The figure shows three views and two pictorial views of one solid part (mm, origin at its lowest corner). Answer the questions. A direction names the side the tool comes from. Coordinates: 2 decimals unless noted, no trailing zeros. Loops run counter-clockwise (first coordinate to the right, second up) from the corner with the lowest first, then second, coordinate; pieces in that order, holes last. Notation, with made-up numbers: (21, 75) -> (38, 75) arc R24 ccw to (38, 90) -> close; hole circle Ø6 at (76, -29). An arc over 180 degrees is marked (long way). Answer as a JSON object with one key per item and string values. Group by question number.
1) Which of the six approach directions +Z, -Z, +X, -X, +Y, -Y give full straight-line access (tool end or side, diameter ignored) to the marked faces 1, 2 and 3?
2) Determine the mould class of the marked faces 4, 5, 6 and 7 for opening direction Z: released by +Z, released by -Z, zero draft, split by the parting line, or undercut.
3) Consider probe 1 along Y at (x, z) = (139.7, 10.75); probe 2 along Y at (x, z) = (139.7, 23.25); probe 3 along Z at (x, y) = (124, 59) (1 decimal). Determine where each line is inside the solid, lowest interval first. Write a range as [from, to].
4) Flat-ended cylindrical pins translate along their axes: P1, Ø19, axis at x = 35.5, z = 81, coming from the -Y side; P2, Ø5, axis at y = 54.5, z = 105.5, coming from the -X side; P3, Ø2, axis at x = 21.5, y = 45.5, coming from the +Z side. Find the tip coordinate at first contact, or state that the pin passes through.
5) Section A-A, the plane y = 38.1 is taken. Count the separate pieces of the cut face and the enclosed holes in it, plus the area to 3 significant figures.
6) Section D-D, the plane z = 79 is taken. Give the vertices of the cut face in (x, y) (1 decimal), plus the area to 3 significant figures.
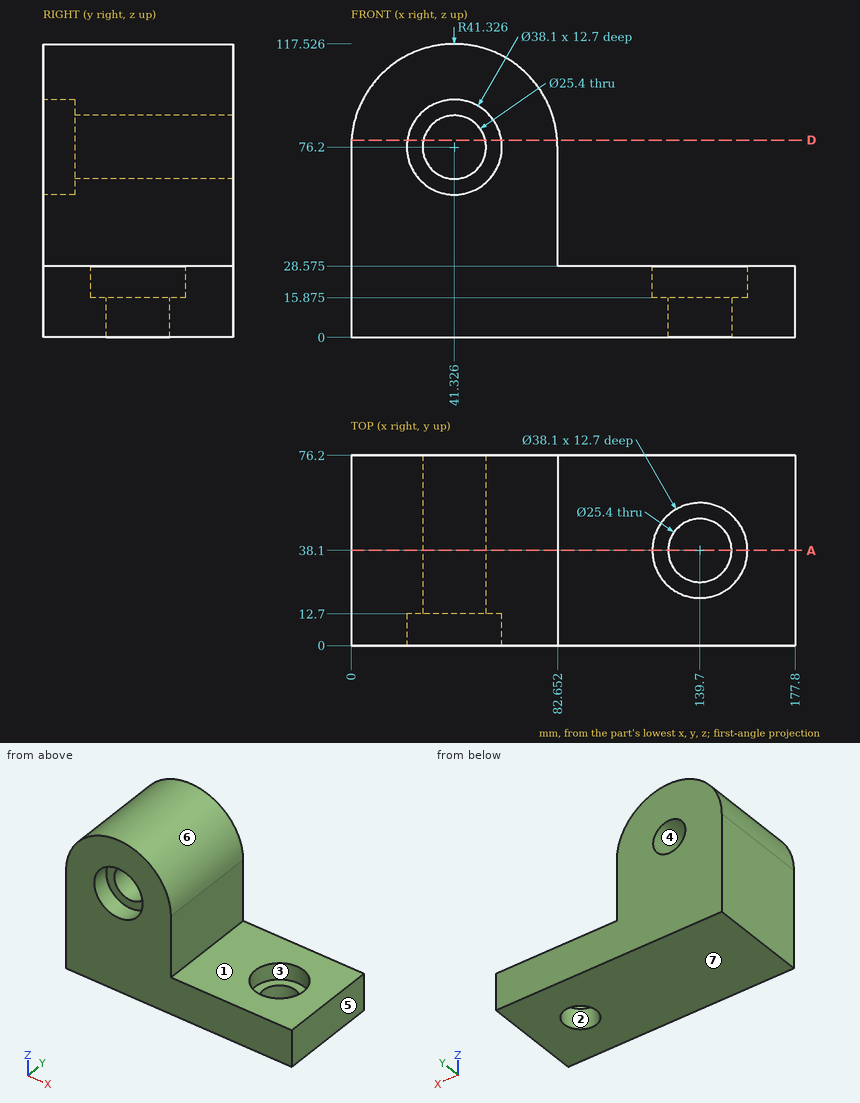
Determined:
{
 "1": {"face 1": "+Z, +X, +Y, -Y", "face 2": "+Z, -Z", "face 3": "+Z"},
 "2": {"face 4": "undercut", "face 5": "zero draft", "face 6": "released by +Z", "face 7": "released by -Z"},
 "3": {"probe 1": "[0, 25.4], [50.8, 76.2]", "probe 2": "[0, 19.05], [57.15, 76.2]", "probe 3": "[0, 28.6]"},
 "4": {"P1": "y = 12.7", "P2": "x = 9.87", "P3": "z = 112.99"},
 "5": {"separate pieces": "2", "enclosed holes": "1", "area": "10,300 mm²"},
 "6": {"outline": "(0.1, 0) -> (22.5, 0) -> (22.5, 12.7) -> (28.9, 12.7) -> (28.9, 76.2) -> (0.1, 76.2) -> close; (53.7, 12.7) -> (60.2, 12.7) -> (60.2, 0) -> (82.6, 0) -> (82.6, 76.2) -> (53.7, 76.2) -> close", "area": "4,230 mm²"}
}
